Read the model definition and answer for the solid it produces. Units are mm, in the model's axes. Face numbers are marked on the shaded views. A direction names the side the tool comes from. Round coordinates to 2 decimals unless told otherwise and drop trailing zeros. Order: outer loops, then holes, each group sorted by start corner. A loop starts at its lowest first (then second) coordinate and runs counter-clockwise, first axis right, second up.
from build123d import *

# Parameters (mm, degrees)
EKSTR_ZYON_NCE2_DEPTH = 5
RADYUS1_R             = 1


with BuildPart() as part:
    # Çizim1 → Ekstrüzyon-İnce2 (new body)
    with BuildSketch(Plane.XY):
        Polygon((82.990542752, -22.308839901), (82.990542752, -33.681351263), (71.790542752, -33.681351263), (71.790542752, -32.681351263), (81.990542752, -32.681351263), (81.990542752, -22.308839901), align=None)
    extrude(amount=EKSTR_ZYON_NCE2_DEPTH)

    # Radyus1
    radyus1_edges = [part.edges().sort_by_distance(p)[0] for p in [
        (81.990542752, -32.681351263, 2.5),
        (82.990542752, -33.681351263, 2.5),
    ]]
    fillet(radyus1_edges, radius=RADYUS1_R)


solid = part.part
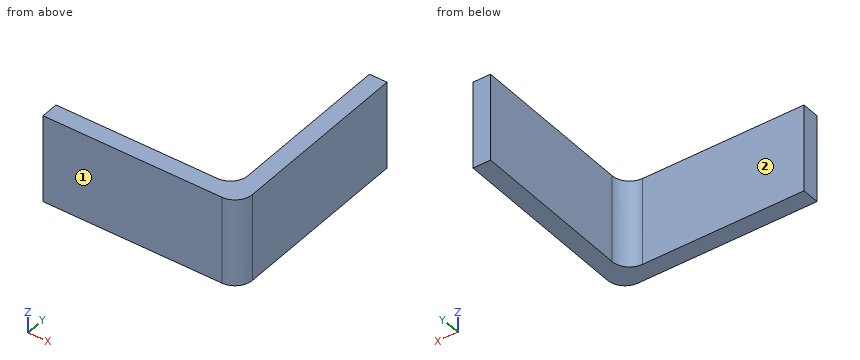
Q1. A cutting plane is placed at C-C, the plane y = -29.25. Give the vertices of the cut face in (x, z), plus the area to 3 significant figures.
Outcome:
outline: (81.99, 0) - (82.99, 0) - (82.99, 5) - (81.99, 5) - close
area: 5.00 mm2
Q2. Straight lines are drawn through the part: probe 1 along Y at (x, z) = (76.25, 1.4); probe 2 along X at (y, z) = (-24, 3.7); probe 3 along Y at (x, z) = (81.5, 2.2). For each, find the intervals that lie inside material, in ascending order.
Outcome:
probe 1: y = -33.68 to -32.68
probe 2: x = 81.99 to 82.99
probe 3: y = -33.68 to -32.54
Q3. A cutting plane is placed at B-B, the plane x = 74. Give the vertices of the cut face in (y, z).
Outcome:
outline: (-33.68, 0) - (-32.68, 0) - (-32.68, 5) - (-33.68, 5) - close
Q4. A cutting plane is placed at A-A, the plane z = 3.05. Give the vertices of the cut face in (x, y), plus the area to 3 significant figures.
Outcome:
outline: (71.79, -33.68) - (81.99, -33.68) arc R1 ccw to (82.99, -32.68) - (82.99, -22.31) - (81.99, -22.31) - (81.99, -31.68) arc R1 cw to (80.99, -32.68) - (71.79, -32.68) - close
area: 21.6 mm2
Q5. For the marked faces 1 and 2, determine the directions among +Z, -Z, +X, -X, +Y, -Y from which every point of the face is accessible in a straight line to the end or side of a thin tool.
Outcome:
face 1: +Z, -Z, +X, -X, -Y
face 2: +Z, -Z, -X, +Y
Q6. Flat-ended cylindrical pins translate along their axes: pin 1 (6 mm diameter, centred on x = 77.5, y = -27, fed in from +Z); pin 2 (1 mm diameter, centred on y = -24.5, z = 0.5, fed in from -X); pin 3 (1.5 mm diameter, centred on x = 76, z = 2, fed in from +Y). Find the tip coordinate at first contact, or state that the pin passes through.
Outcome:
pin 1: passes through
pin 2: stops at x = 81.99
pin 3: stops at y = -32.68
